The model under review builds one solid part; all positions refer to its coordinate system, in mm. Face numbers are marked on the shaded views. A direction names the side the tool comes from. Round coordinates to 2 decimals unless told otherwise and drop trailing zeros. Order: outer loops, then holes, each group sorted by start corner. A loop starts at its lowest first (then second) coordinate and runs counter-clockwise, first axis right, second up.
1) Consider section C-C (z = 11). Give the boundary of the cut face in (x, y).
2) Machinability: for the marked faces 4, 5, 6, 7 and 8, which of the approach directions +Z, -Z, +X, -X, +Y, -Y give a long, thin tool a straight path to every point of the face, cutting with its end or side? Answer none if there is none.
3) Consider section B-B (z = 28.5). Give the boundary of the cut face in (x, y), then the cut area to 3 significant figures.
4) To check wall thickness, follow L1, parallel to Y at x = -30, z = 4.5; L2, parallel to Y at x = 23, z = 21.5; L3, parallel to Z at x = -39, y = 9. State the ranges of each line that lie inside material, in increasing order.
5) Consider section A-A (x = -24). Give the boundary of the cut face in (y, z).
6) Mouldability with a two-part tool opening along X and no side actions: class the marked faces 1, 2 and 3 as pulls with the +X half, pulls with the -X half, needs draft (parallel to the pull), parting line crosses it, or undercut.
7) Clearance check with flat-ended pins moving along their axes: P1, Ø6, axis at x = -3, z = 12, coming from the +Y side; P2, Ø4, axis at x = -11, z = 57, coming from the -Y side; P3, Ø18, axis at x = -16.5, y = 52, coming from the +Z side. State where each tip first meets the part, or that it passes through.
8) Consider section D-D (x = 0). Give the boundary of the cut face in (y, z).
from build123d import *

# Parameters (mm, degrees)
SKETCH_1_R          = 10
EXTRUDE_1_DEPTH     = 20
FILLET_1_R          = 20
EXTRUDE_2_DEPTH     = 50
SKETCH_3_W          = 100
SKETCH_3_H          = 20
EXTRUDE_3_DEPTH     = 35
FILLET_2_R          = 5
CUT_EXTRUDE_START   = -50
CUT_EXTRUDE_1_DEPTH = 50


with BuildPart() as part:
    # 草圖1 → 填料-伸長1 (new body)
    with BuildSketch(Plane.XY):
        Polygon((-50, 80), (-10, 80), (-10, 50), (10, 50), (10, 80), (50, 80), (50, 0), (-50, 0), align=None)
        with Locations((-30, 60)):
            Circle(SKETCH_1_R, mode=Mode.SUBTRACT)
        with Locations((30, 60)):
            Circle(SKETCH_1_R, mode=Mode.SUBTRACT)
    extrude(amount=EXTRUDE_1_DEPTH)

    # 圓角1
    fillet_1_edges = [part.edges().sort_by_distance(p)[0] for p in [
        (-50, 80, 10),
        (50, 80, 10),
    ]]
    fillet(fillet_1_edges, radius=FILLET_1_R)

    # 草圖2 → 填料-伸長2 (add)
    with BuildSketch(Plane.XY.offset(20)):
        with BuildLine():
            ThreePointArc((-20, 0), (0, 20), (20, 0))
            Line((20, 0), (30, 0))
            ThreePointArc((30, 0), (0, 30), (-30, 0))
            Line((-30, 0), (-20, 0))
        make_face()
    extrude(amount=EXTRUDE_2_DEPTH)

    # 草圖3 → 填料-伸長3 (add)
    with BuildSketch(Plane.XY.offset(20)):
        with Locations((0, 10)):
            Rectangle(SKETCH_3_W, SKETCH_3_H)
    extrude(amount=EXTRUDE_3_DEPTH)

    # 圓角2
    fillet_2_edges = [part.edges().sort_by_distance(p)[0] for p in [
        (50, 10, 55),
        (-50, 10, 55),
    ]]
    fillet(fillet_2_edges, radius=FILLET_2_R)

    # 草圖4 → 除料-伸長1 (cut)
    with BuildSketch(Plane.XY.offset(70).offset(CUT_EXTRUDE_START)):
        with BuildLine():
            Line((-20, 0), (20, 0))
            ThreePointArc((20, 0), (0, 20), (-20, 0))
        make_face()
    extrude(amount=CUT_EXTRUDE_1_DEPTH, mode=Mode.SUBTRACT)


solid = part.part
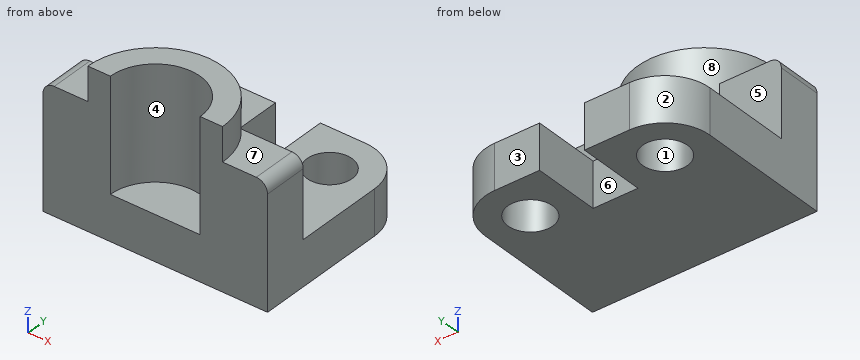
Answer below:
1. outline: (-50, 0) - (50, 0) - (50, 60) arc R20 ccw to (30, 80) - (10, 80) - (10, 50) - (-10, 50) - (-10, 80) - (-30, 80) arc R20 ccw to (-50, 60) - close; hole circle Ø20 at (-30, 60); hole circle Ø20 at (30, 60)
2. face 4: +Z, -Y
2. face 5: +Z, -X, +Y
2. face 6: +Z, -Z, +Y
2. face 7: +Z, +X, +Y
2. face 8: +Z, +Y
3. outline: (-50, 0) - (-20, 0) arc R20 cw to (20, 0) - (50, 0) - (50, 20) - (22.36, 20) arc R30 ccw to (-22.36, 20) - (-50, 20) - close
3. area: 1,680 mm2
4. L1: y = 0 to 50, 70 to 80
4. L2: y = 0 to 20
4. L3: z = 0 to 55
5. outline: (0, 0) - (52, 0) - (52, 20) - (20, 20) - (20, 55) - (18, 55) - (18, 70) - (0, 70) - close; (68, 0) - (80, 0) - (80, 20) - (68, 20) - close
6. face 1: undercut
6. face 2: pulls with the -X half
6. face 3: needs draft
7. P1: stops at y = 50
7. P2: stops at y = 15.2
7. P3: stops at z = 20
8. outline: (0, 0) - (50, 0) - (50, 20) - (30, 20) - (30, 70) - (20, 70) - (20, 20) - (0, 20) - close
